```python
from build123d import *

# Parameters (mm, degrees)
F0_R     = 10.9855
F1_DEPTH = 6.35
F2_R     = 2.54


with BuildPart() as f1:
    # F0 (on Top) → F1 (new body)
    with BuildSketch(Plane.XY):
        with BuildLine():
            ThreePointArc((-16.29171875, -7.1209760687), (-17.4039529903, -3.6374194579), (-17.78, 0))
            ThreePointArc((-17.78, 0), (-17.4039529903, 3.6374194579), (-16.29171875, 7.1209760687))
            ThreePointArc((-16.29171875, 7.1209760687), (-18.8020162617, 10.7536189633), (-22.2158041159, 13.554286827))
            ThreePointArc((-22.2158041159, 13.554286827), (-46.355, 0), (-22.2158041159, -13.554286827))
            ThreePointArc((-22.2158041159, -13.554286827), (-18.8020162617, -10.7536189633), (-16.29171875, -7.1209760687))
        make_face()
        with Locations((-30.48, 0)):
            Circle(F0_R, mode=Mode.SUBTRACT)
        with BuildLine():
            ThreePointArc((-22.2158041159, 13.554286827), (-18.8020162617, 10.7536189633), (-16.29171875, 7.1209760687))
            ThreePointArc((-16.29171875, 7.1209760687), (-13.9800556545, 10.9857382044), (-10.7715482955, 14.1457466158))
            ThreePointArc((-10.7715482955, 14.1457466158), (-16.4023314736, 12.0825720001), (-22.2158041159, 13.554286827))
        make_face()
        with BuildLine():
            ThreePointArc((-10.7715482955, -14.1457466158), (-13.9800556545, -10.9857382044), (-16.29171875, -7.1209760687))
            ThreePointArc((-16.29171875, -7.1209760687), (-18.8020162617, -10.7536189633), (-22.2158041159, -13.554286827))
            ThreePointArc((-22.2158041159, -13.554286827), (-16.4023314736, -12.0825720001), (-10.7715482955, -14.1457466158))
        make_face()
        with BuildLine():
            Line((14.605, 0), (10.9855, 0))
            ThreePointArc((10.9855, 0), (0, -10.9855), (-10.9855, 0))
            Line((-10.9855, 0), (-14.605, 0))
            ThreePointArc((-14.605, 0), (-15.032434013, -3.6590067065), (-16.29171875, -7.1209760687))
            ThreePointArc((-16.29171875, -7.1209760687), (-13.9800556545, -10.9857382044), (-10.7715482955, -14.1457466158))
            ThreePointArc((-10.7715482955, -14.1457466158), (0, -17.78), (10.7715482955, -14.1457466158))
            ThreePointArc((10.7715482955, -14.1457466158), (13.9800556545, -10.9857382044), (16.29171875, -7.1209760687))
            ThreePointArc((16.29171875, -7.1209760687), (15.032434013, -3.6590067065), (14.605, 0))
        make_face()
        with BuildLine():
            ThreePointArc((-10.9855, 0), (0, 10.9855), (10.9855, 0))
            Line((10.9855, 0), (14.605, 0))
            ThreePointArc((14.605, 0), (15.032434013, 3.6590067065), (16.29171875, 7.1209760687))
            ThreePointArc((16.29171875, 7.1209760687), (13.9800556545, 10.9857382044), (10.7715482955, 14.1457466158))
            ThreePointArc((10.7715482955, 14.1457466158), (0, 17.78), (-10.7715482955, 14.1457466158))
            ThreePointArc((-10.7715482955, 14.1457466158), (-13.9800556545, 10.9857382044), (-16.29171875, 7.1209760687))
            ThreePointArc((-16.29171875, 7.1209760687), (-15.032434013, 3.6590067065), (-14.605, 0))
            Line((-14.605, 0), (-10.9855, 0))
        make_face()
        with BuildLine():
            ThreePointArc((10.7715482955, 14.1457466158), (13.9800556545, 10.9857382044), (16.29171875, 7.1209760687))
            ThreePointArc((16.29171875, 7.1209760687), (18.8020162617, 10.7536189633), (22.2158041159, 13.554286827))
            ThreePointArc((22.2158041159, 13.554286827), (16.4023314736, 12.0825720001), (10.7715482955, 14.1457466158))
        make_face()
        with BuildLine():
            ThreePointArc((22.2158041159, -13.554286827), (18.8020162617, -10.7536189633), (16.29171875, -7.1209760687))
            ThreePointArc((16.29171875, -7.1209760687), (13.9800556545, -10.9857382044), (10.7715482955, -14.1457466158))
            ThreePointArc((10.7715482955, -14.1457466158), (16.4023314736, -12.0825720001), (22.2158041159, -13.554286827))
        make_face()
        with BuildLine():
            ThreePointArc((16.29171875, 7.1209760687), (17.4039529903, 3.6374194579), (17.78, 0))
            ThreePointArc((17.78, 0), (17.4039529903, -3.6374194579), (16.29171875, -7.1209760687))
            ThreePointArc((16.29171875, -7.1209760687), (18.8020162617, -10.7536189633), (22.2158041159, -13.554286827))
            ThreePointArc((22.2158041159, -13.554286827), (38.2524357617, -13.8421409952), (46.355, 0))
            ThreePointArc((46.355, 0), (38.2524357617, 13.8421409952), (22.2158041159, 13.554286827))
            ThreePointArc((22.2158041159, 13.554286827), (18.8020162617, 10.7536189633), (16.29171875, 7.1209760687))
        make_face()
        with BuildLine():
            ThreePointArc((41.4655, 0), (30.48, -10.9855), (19.4945, 0))
            ThreePointArc((19.4945, 0), (30.48, 10.9855), (41.4655, 0))
        make_face(mode=Mode.SUBTRACT)
    extrude(amount=F1_DEPTH)

    # F2
    f2_edges = [f1.edges().sort_by_distance(p)[0] for p in [
        (-46.355, 0, 6.35),
        (-16.402331, 12.082572, 6.35),
        (0, 17.78, 6.35),
        (16.402331, 12.082572, 6.35),
        (46.355, 0, 6.35),
        (16.402331, -12.082572, 6.35),
        (0, -17.78, 6.35),
        (-16.402331, -12.082572, 6.35),
        (-46.355, 0, 0),
        (-16.402331, -12.082572, 0),
        (0, -17.78, 0),
        (-16.402331, 12.082572, 0),
        (0, 17.78, 0),
        (16.402331, -12.082572, 0),
        (46.355, 0, 0),
        (16.402331, 12.082572, 0),
    ]]
    fillet(f2_edges, radius=F2_R)


solid = f1.part
```
Could you check a few things on this model? Use its own coordinates, in mm. Round coordinates to 2 decimals unless told otherwise and drop trailing zeros. Loops run counter-clockwise (first coordinate to the right, second up) from the corner with the lowest first, then second, coordinate; pieces in that order, holes last. Notation, with made-up numbers: (-3, 45.25) -> (28, 45.25) arc R12 ccw to (28, 58.25) -> close; hole circle Ø7 at (43, -37.5). An arc over 180 degrees is marked (long way). One line per question, with ' | ' between items.
(1) Thinking about a two-plate mould opening in Y: for faces 1 (the face through (0.16, 17.78, 3.17)), 2 (the face through (-10.48, 3.3, 3.13)), 3 (the face through (10, -6, 0)), which applies, released by +Y, released by -Y, zero draft, split by the parting line, or undercut?
Model answer:
face 1: released by +Y | face 2: undercut | face 3: zero draft
(2) For pin 1 Ø1 at (x, y) = (15.5, -10.5) entering from +Z; pin 2 Ø6 at (x, y) = (-32, -11.5) entering from -Z; pin 3 Ø1 at (y, z) = (6.5, 5) entering from +X, each with a flat end and sliding along its axis, tell me the tip position at first contact or that it passes through.
Model answer:
pin 1: stops at z = 6.32 | pin 2: stops at z = 0 | pin 3: stops at x = 44.96
(3) If we section it at A-A on x = 0: List the corners of the cut face in (y, z) for me, and give its area (3 significant figures).
Model answer:
outline: (-17.78, 2.54) arc R2.54 ccw to (-15.24, 0) -> (-10.99, 0) -> (-10.99, 6.35) -> (-15.24, 6.35) arc R2.54 ccw to (-17.78, 3.81) -> close; (10.99, 0) -> (15.24, 0) arc R2.54 ccw to (17.78, 2.54) -> (17.78, 3.81) arc R2.54 ccw to (15.24, 6.35) -> (10.99, 6.35) -> close | area: 80.8 mm^2
(4) If I drill on probe 1 along Y at (x, z) = (0.5, 3.75); probe 2 along X at (y, z) = (-3, 4.5); probe 3 along X at (y, z) = (2.5, 5), over which ranges is the centre line in solid material (lowest first)?
Model answer:
probe 1: y = -17.77 to -10.97, 10.97 to 17.77 | probe 2: x = -45.97 to -41.05, -19.91 to -17.53, -14.89 to -10.57, 10.57 to 14.89, 17.53 to 19.91, 41.05 to 45.97 | probe 3: x = -45.86 to -41.18, -19.78 to -17.6, -14.8 to -10.7, 10.7 to 14.8, 17.6 to 19.78, 41.18 to 45.86
(5) If we section it at B-B on z = 4.75: Count the separate pieces of the cut face and the enclosed holes in it, and give its area (3 significant figures).
Model answer:
separate pieces: 1 | enclosed holes: 5 | area: 1,350 mm^2
